Can you work these out from the model? Positions are in its coordinate system, mm. A direction names the side the tool comes from. Coordinates: 2 decimals unless noted, no trailing zeros. Loops run counter-clockwise (first coordinate to the right, second up) from the corner with the lowest first, then second, coordinate; pieces in that order, holes last.
```python
from build123d import *

# Parameters (mm, degrees)
SKETCH_1_W          = 10
SKETCH_1_H          = 10
SKETCH_1_W_2        = 8
SKETCH_1_H_2        = 8
EXTRUDE_1_DEPTH     = 50
SKETCH_2_R          = 4
SKETCH_2_R_2        = 1.6
CUT_EXTRUDE_1_DEPTH = 52.961524227
CUT_EXTRUDE_2_REACH = 53.962
SKETCH_4_R          = 2.6
SKETCH_5_R          = 1.6
CUT_EXTRUDE_3_DEPTH = 52.961524227


with BuildPart() as part:
    # ｽｹｯﾁ1 → 押し出し-薄板1 (new body)
    with BuildSketch(Plane.XY):
        with Locations((5, 5)):
            Rectangle(SKETCH_1_W, SKETCH_1_H)
        with Locations((5, 5)):
            Rectangle(SKETCH_1_W_2, SKETCH_1_H_2, mode=Mode.SUBTRACT)
    extrude(amount=EXTRUDE_1_DEPTH)

    # ｽｹｯﾁ2 → ｶｯﾄ - 押し出し1 (cut, through all)
    with BuildSketch(Plane(origin=(0, 10, 0), x_dir=(1, 0, 0), z_dir=(0, 1, 0))):
        with Locations(Location((5, -10.5, 0), (0, 0, 270))):
            Circle(SKETCH_2_R)
        with Locations(Location((5, -19.5, 0), (0, 0, 270))):
            Circle(SKETCH_2_R_2)
    extrude(amount=-CUT_EXTRUDE_1_DEPTH, mode=Mode.SUBTRACT)

    # ｽｹｯﾁ4 → ｶｯﾄ - 押し出し2 (cut, up to next)
    with BuildSketch(Plane.XZ, mode=Mode.PRIVATE) as cut_extrude_2_sk1:
        with Locations(Location((5, 19.5, 0), (0, 0, 270))):
            Circle(SKETCH_4_R)
    cut_extrude_2_tool1 = extrude(cut_extrude_2_sk1.sketch, amount=-CUT_EXTRUDE_2_REACH, mode=Mode.PRIVATE) & part.part
    add(cut_extrude_2_tool1.solids().sort_by_distance((5, 0, 19.5))[0], mode=Mode.SUBTRACT)

    # ｽｹｯﾁ5 → ｶｯﾄ - 押し出し3 (cut, through all)
    with BuildSketch(Plane(origin=(10, 0, 0), x_dir=(0, 0, -1), z_dir=(1, 0, 0))):
        with Locations(Location((-45, 5, 0), (0, 0, 90))):
            Circle(SKETCH_5_R)
    extrude(amount=-CUT_EXTRUDE_3_DEPTH, mode=Mode.SUBTRACT)


solid = part.part
```
(1) I want a section at D-D on y = 2.75. Write out the boundary of the cut face in (x, z).
Check values:
outline: (0, 0) - (1, 0) - (1, 50) - (0, 50) - close; (9, 0) - (10, 0) - (10, 50) - (9, 50) - close
(2) I'm going to push flat-ended pins straight in: pin 1 (1.5 mm diameter, centred on x = 3.5, y = 1.5, fed in from +Z); pin 2 (4 mm diameter, centred on x = 5, z = 19.5, fed in from -Y). Where does each tip first touch, or does it pass through?
Check values:
pin 1: stops at z = 50
pin 2: stops at y = 9
(3) If I drill on probe 1 along Y at (x, z) = (8.75, 18.5); probe 2 along X at (y, z) = (0.75, 19.5), over which ranges is the centre line in solid material (lowest first)?
Check values:
probe 1: y = 0 to 1, 9 to 10
probe 2: x = 0 to 2.4, 7.6 to 10
(4) Which directions (+Z, -Z, +X, -X, +Y, -Y) give clear straight access to the entire face, cutting with the end or side of a thin tool? Please do faces 5 (the cylindrical face through (9.51, 5.74, 43.58)), 6 (the cylindrical face through (5.78, 0.49, 17.02)), 7 (the flat face through (5, 9, 30)).
Check values:
face 5: +X, -X
face 6: -Y
face 7: +Z, -Z
(5) I want a section at C-C on x = 5. Write out the boundary of the cut face in (y, z).
Check values:
outline: (0, 0) - (1, 0) - (1, 6.5) - (0, 6.5) - close; (0, 14.5) - (1, 14.5) - (1, 16.9) - (0, 16.9) - close; (0, 22.1) - (1, 22.1) - (1, 50) - (0, 50) - close; (9, 0) - (10, 0) - (10, 6.5) - (9, 6.5) - close; (9, 14.5) - (10, 14.5) - (10, 17.9) - (9, 17.9) - close; (9, 21.1) - (10, 21.1) - (10, 50) - (9, 50) - close
(6) I want a section at A-A on z = 19.5. Write out the boundary of the cut face in (x, y).
Check values:
outline: (0, 0) - (2.4, 0) - (2.4, 1) - (1, 1) - (1, 9) - (3.4, 9) - (3.4, 10) - (0, 10) - close; (6.6, 9) - (9, 9) - (9, 1) - (7.6, 1) - (7.6, 0) - (10, 0) - (10, 10) - (6.6, 10) - close
(7) I want a section at B-B on y = 5. Write out the boundary of the cut face in (x, z), then the cut area to 3 significant figures.
Check values:
outline: (0, 0) - (1, 0) - (1, 43.4) - (0, 43.4) - close; (0, 46.6) - (1, 46.6) - (1, 50) - (0, 50) - close; (9, 0) - (10, 0) - (10, 43.4) - (9, 43.4) - close; (9, 46.6) - (10, 46.6) - (10, 50) - (9, 50) - close
area: 93.6 mm2
(8) If we mould it in two halves opening along Z, with no side actions, what happens to faces 1 (the cylindrical face through (0.51, 5.74, 43.58)), 2 (the flat face through (5, 10, 25)), 3 (the flat face through (0.5, 5.1, 0)), 4 (the flat face through (0.5, 5.1, 50))? For each: released by +Z, released by -Z, zero draft, split by the parting line, or undercut.
Check values:
face 1: undercut
face 2: zero draft
face 3: released by -Z
face 4: released by +Z
